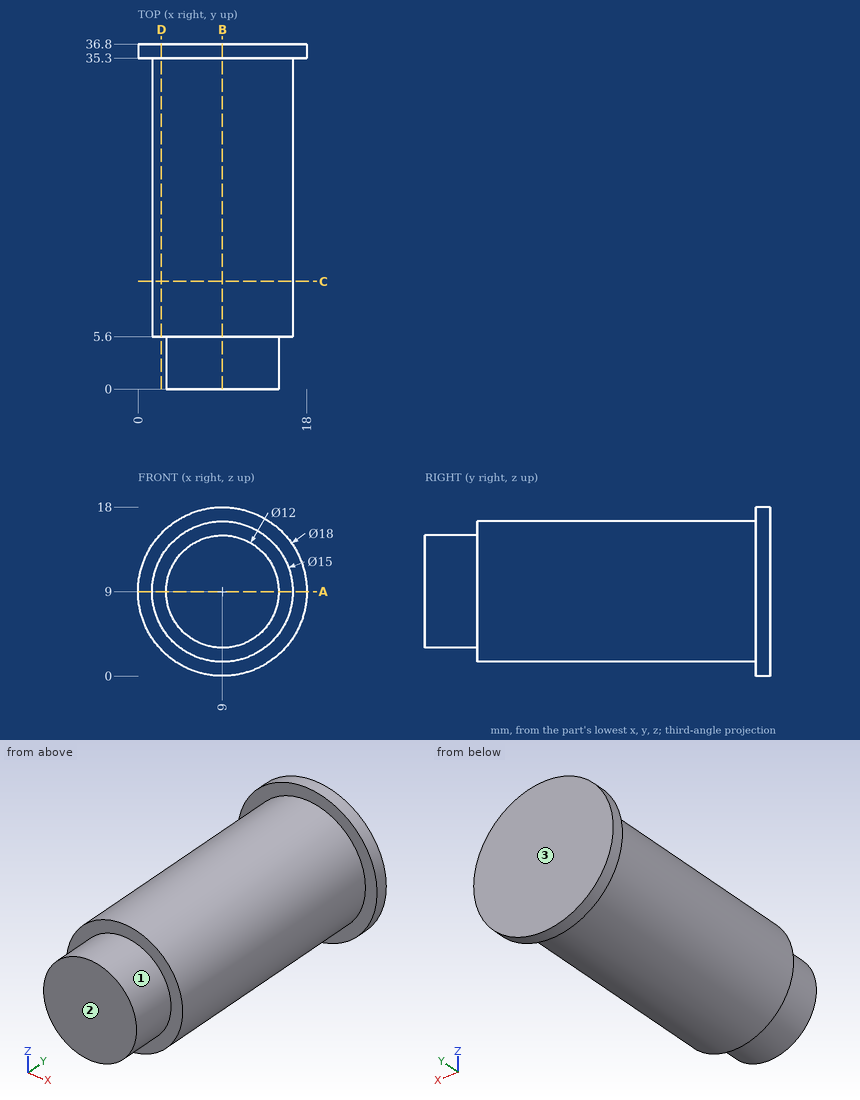
Design review of the part shown in the three views and the two pictorial views. Dimensions are in mm from the part's minimum x, y and z. Round coordinates to 2 decimals unless told otherwise and drop trailing zeros. Loops run counter-clockwise (first coordinate to the right, second up) from the corner with the lowest first, then second, coordinate; pieces in that order, holes last. Notation, with made-up numbers: M -33.75,-20.5 L 5.25,-20.5 A19 ccw 5.25,-6.5 Z; hole C 32,-33.5 d3. An arc over 180 degrees is marked long. Answer as a JSON object with one key per item and string values.
Item 1: We need section D-D, the plane x = 2.5. State the section outline as (y, z) points, and give its area (3 significant figures).
Check sheet entries:
{"outline": "M 5.6,5.26 L 35.3,5.26 L 35.3,2.78 L 36.8,2.78 L 36.8,15.22 L 35.3,15.22 L 35.3,12.74 L 5.6,12.74 Z", "area": "241 mm2"}
Item 2: We need section B-B, the plane x = 9. State the section outline as (y, z) points, and give its area (3 significant figures).
Check sheet entries:
{"outline": "M 0,3 L 5.6,3 L 5.6,1.5 L 35.3,1.5 L 35.3,0 L 36.8,0 L 36.8,18 L 35.3,18 L 35.3,16.5 L 5.6,16.5 L 5.6,15 L 0,15 Z", "area": "540 mm2"}
Item 3: We need section C-C, the plane y = 11.5. State the section outline as (x, z) points, and give its area (3 significant figures).
Check sheet entries:
{"outline": "C 9,9 d15", "area": "177 mm2"}
Item 4: The part is to be moulded in two halves that separate along Y. For the marked faces 1, 2 and 3, say which applies: +Y half, -Y half, draft (parallel to the pull), parting line (faces both ways), or undercut.
Check sheet entries:
{"face 1": "draft", "face 2": "-Y half", "face 3": "+Y half"}
Item 5: We need section A-A, the plane z = 9. State the section outline as (x, y) points, and give its area (3 significant figures).
Check sheet entries:
{"outline": "M 0,35.3 L 1.5,35.3 L 1.5,5.6 L 3,5.6 L 3,0 L 15,0 L 15,5.6 L 16.5,5.6 L 16.5,35.3 L 18,35.3 L 18,36.8 L 0,36.8 Z", "area": "540 mm2"}
Item 6: Clearance check with flat-ended pins moving along their axes: P1, Ø4, axis at x = 15.5, y = 21, coming from the +Z side; P2, Ø4, axis at x = 15.5, z = 2, coming from the -Y side; P3, Ø6, axis at x = 7.5, y = 6, coming from the -Z side. State where each tip first meets the part, or that it passes through.
Check sheet entries:
{"P1": "z = 15", "P2": "y = 35.3", "P3": "z = 1.5"}
Item 7: For line 1 along Y through (x, z) = (16.75, 6.75); line 2 along X through (y, z) = (23.5, 13.5); line 3 along X through (y, z) = (15, 9), list the stretches that pass through material, from the lowest coordinate up.
Check sheet entries:
{"line 1": "35.3 to 36.8", "line 2": "3 to 15", "line 3": "1.5 to 16.5"}
